Part model, mm, in its own coordinate system. A direction names the side the tool comes from. Give positions to 0.01 mm unless a question says otherwise; leave off trailing zeros. Order: outer loops, then holes, each group sorted by start corner. A loop starts at its lowest first (then second) coordinate and runs counter-clockwise, first axis right, second up. Notation, with made-up numbers: (-18.75, 87.25) - (25.25, 87.25) arc R19 cw to (25.25, 113.25) - close; hole circle Ø9 at (47.25, 42.5). An arc over 180 degrees is marked (long way). One line per item, written item: value.
```python
from build123d import *

# Parameters (mm, degrees)
F1_DEPTH    = 50.8
F4_DEPTH    = 3.175
F5_T4_DEPTH = 13.5737083661
F5_T9_DEPTH = 13.5737083661
F6_R        = 1.397
F7_T1_DEPTH = 26.6857916153
F7_T4_ANGLE = 90
F7_T6_ANGLE = 90


# Not quite as in the source:
# - a fillet or chamfer that OpenCascade refuses, or shapes differently, is made with other operations: its cross-section is extruded or revolved along the edge and cut away or added


with BuildPart() as f1:
    # F0 (on Top) → F1 (new body)
    with BuildSketch(Plane.XY):
        Polygon((16.83116441, 6.3822651147), (-9.8546272053, 6.3822651147), (-9.8546272053, -2.4114359531), (-9.1195573698, -0.8609411879), (-7.5529336119, 0.5598957894), (-4.6044890144, 2.2076013963), (0.7639104889, 3.3147196292), (6.2126267158, 3.3147196292), (11.5810262191, 2.2076013963), (14.5294708166, 0.5598957894), (16.0960945745, -0.8609411879), (16.83116441, -2.4114359531), align=None)
    extrude(amount=F1_DEPTH)

    # F3 (on face) → F4 (join)
    with BuildSketch(Plane.XY.offset(50.8)):
        Polygon((11.6162686024, 6.3822651147), (-4.6397313976, 6.3822651147), (-4.6397313976, 2.2003334042), (0.7639104889, 3.3147196292), (6.2126267158, 3.3147196292), (11.6162686024, 2.2003334042), align=None)
    extrude(amount=F4_DEPTH)

    # F5: fillet of radius 3.81 on 2 edges, made by hand


with BuildPart() as f5_tool2:
    # F5_s3 → F5_t4 (new body)
    with BuildSketch(Plane.XZ.offset(7.1914432514)):
        with BuildLine():
            ThreePointArc((15.3729792646, 50.8), (12.9136348398, 51.7000644337), (11.6162686024, 53.975))
            Line((11.6162686024, 53.975), (11.6162686024, 50.8))
            Line((11.6162686024, 50.8), (15.3729792646, 50.8))
        make_face()
    extrude(amount=-F5_T4_DEPTH)

    split(bisect_by=Plane(origin=(0.9091488864, 4.4084491475, 0), x_dir=(0, 0, 1), z_dir=(0.2019783567, 0.9793899854, 0)), keep=Keep.TOP)


with BuildPart() as f1_1:
    add(f1.part)

    # F5_t1: union F5_tool2
    add(f5_tool2.part)


with BuildPart() as f5_tool7:
    # F5_s8 → F5_t9 (new body)
    with BuildSketch(Plane.XZ.offset(-6.3822651147)):
        with BuildLine():
            ThreePointArc((-8.3964420599, 50.8), (-5.9370976351, 51.7000644337), (-4.6397313976, 53.975))
            Line((-4.6397313976, 53.975), (-4.6397313976, 50.8))
            Line((-4.6397313976, 50.8), (-8.3964420599, 50.8))
        make_face()
    extrude(amount=F5_T9_DEPTH)

    split(bisect_by=Plane(origin=(-0.624539261, 3.0283813951, 0), x_dir=(0, 0, 1), z_dir=(-0.2019783567, 0.9793899854, 0)), keep=Keep.TOP)


with BuildPart() as f1_2:
    add(f1_1.part)

    # F5_t6: union F5_tool7
    add(f5_tool7.part)

    # F6
    f6_edges = [f1_2.edges().sort_by_distance(p)[0] for p in [
        (-9.854627, 1.985415, 50.8),
        (16.831164, 1.985415, 50.8),
        (16.831164, 1.985415, 0),
        (-9.854627, 1.985415, 0),
        (16.831164, 6.382265, 25.4),
        (-9.854627, 6.382265, 25.4),
    ]]
    fillet(f6_edges, radius=F6_R)

    # F7: fillet of radius 2.54 on 1 edges, made by hand

    # F7_s2 → F7_t1 (cut)
    with BuildSketch(Plane.YZ.offset(-9.8546272053)):
        with BuildLine():
            ThreePointArc((6.3822651147, 2.54), (5.6383163389, 0.7439487758), (3.8422651147, 0))
            Line((3.8422651147, 0), (6.3822651147, 0))
            Line((6.3822651147, 0), (6.3822651147, 2.54))
        make_face()
    extrude(amount=F7_T1_DEPTH, mode=Mode.SUBTRACT)

    # F7_s3 → F7_t4 (revolve, cut)
    with BuildSketch(Plane.XZ.offset(-3.8422651147)):
        with BuildLine():
            ThreePointArc((16.83116441, 1.397), (16.4219925833, 0.4091718267), (15.43416441, 0))
            Line((15.43416441, 0), (16.83116441, 0))
            Line((16.83116441, 0), (16.83116441, 1.397))
        make_face()
    revolve(axis=Axis((16.83116441, 3.8422651147, 2.54), (1, 0, 0)), revolution_arc=F7_T4_ANGLE, mode=Mode.SUBTRACT)

    # F7_s5 → F7_t6 (revolve, cut)
    with BuildSketch(Plane.XY.offset(2.54)):
        with BuildLine():
            ThreePointArc((-9.8546272053, 4.9852651147), (-9.4454553786, 5.973093288), (-8.4576272053, 6.3822651147))
            Line((-8.4576272053, 6.3822651147), (-9.8546272053, 6.3822651147))
            Line((-9.8546272053, 6.3822651147), (-9.8546272053, 4.9852651147))
        make_face()
    revolve(axis=Axis((-9.8546272053, 3.8422651147, 2.54), (-1, 0, 0)), revolution_arc=F7_T6_ANGLE, mode=Mode.SUBTRACT)


solid = f1_2.part
```
1) Mould opens along X. For faces 4 (the cylindrical face through (12.94, 3.87, 51.68)), 5 (the flat face through (-9.492, -1.647, 25.047)), 6 (the cylindrical face through (-5.966, 3.939, 51.676)) say: released by +X, released by -X, zero draft, split by the parting line, or undercut.
Outcome:
face 4: released by +X
face 5: undercut
face 6: released by -X
2) Drill centre lines: line 1 along Y through (x, z) = (4.75, 46); line 2 along X through (y, z) = (-0.5, 37.5); line 3 along X through (y, z) = (0, 8.5). Where is each one in solid material? Low to high. Write a range as from..to.
Outcome:
line 1: y = 3.31..6.38
line 2: x = -9.85..-8.72, 15.7..16.83
line 3: x = -9.85..-8.17, 15.15..16.83
3) Pin check, flat tips, straight feed: pin 1 (1.9 mm diameter, centred on x = 12.5, y = 3, fed in from +Z) (3 decimals); pin 2 (2 mm diameter, centred on x = 11.5, z = 25, fed in from -Y); pin 3 (1.6 mm diameter, centred on x = 4.5, z = 20.5, fed in from -Y); pin 4 (1 mm diameter, centred on x = 0.5, z = 48.5, fed in from -Y). Stop position of each tip, or through.
Outcome:
pin 1: stops at z = 53.975
pin 2: stops at y = 1.69
pin 3: stops at y = 3.31
pin 4: stops at y = 3.16
4) Cut at B-B, the plane x = 13.5. Give the cut face in (y, z), then the cut area to 3 significant figures.
Outcome:
outline: (1.14, 0) - (3.84, 0) arc R2.54 ccw to (6.38, 2.54) - (6.38, 51.29) - (1.81, 51.29) - (1.81, 50.8) - (1.14, 50.8) - close
area: 267 mm^2
5) Which spindle directions (+Z, -Z, +X, -X, +Y, -Y) get a long thin tool onto all of the face, cutting with end or side? Do faces 1 (the cylindrical face through (16.41, 1.45, 0.4)), 2 (the flat face through (-7.3, 1.1, 50.8)), 3 (the flat face through (13.03, 1.4, 25.04)). Say none if no direction does.
Outcome:
face 1: -Z, +X, +Y, -Y
face 2: +Z, -Y
face 3: +Z, -Z, -Y
6) Cut at A-A, the plane z = 45.5. Give the cut face in (x, y).
Outcome:
outline: (-9.85, -2.41) - (-9.12, -0.86) - (-7.55, 0.56) - (-4.6, 2.21) - (0.76, 3.31) - (6.21, 3.31) - (11.58, 2.21) - (14.53, 0.56) - (16.1, -0.86) - (16.83, -2.41) - (16.83, 4.99) arc R1.4 ccw to (15.43, 6.38) - (-8.46, 6.38) arc R1.4 ccw to (-9.85, 4.99) - close
7) Cut at C-C, the plane x = -6. Give the cut face in (y, z), then the cut area to 3 significant figures.
Outcome:
outline: (1.43, 0) - (3.84, 0) arc R2.54 ccw to (6.38, 2.54) - (6.38, 51.65) - (1.92, 51.65) - (1.92, 50.8) - (1.43, 50.8) - close
area: 254 mm^2
8) Cut at D-D, the plane x = 7.75. Give the cut face in (y, z) (3 decimals).
Outcome:
outline: (2.998, 0) - (3.842, 0) arc R2.54 ccw to (6.382, 2.54) - (6.382, 53.975) - (2.998, 53.975) - close
